Design review of the part built by this model. Coordinates are the model's own, in mm. A direction names the side the tool comes from. Round coordinates to 2 decimals unless told otherwise and drop trailing zeros. Loops run counter-clockwise (first coordinate to the right, second up) from the corner with the lowest first, then second, coordinate; pieces in that order, holes last. Notation, with made-up numbers: (59.25, 39) - (76.25, 39) arc R7 cw to (76.25, 52) - close; hole circle Ø2 at (60, 12). An arc over 180 degrees is marked (long way). One line per question, with ' | ' between items. Start each with the question number.
from build123d import *

# Parameters (mm, degrees)
CROQUIS1_W              = 5.15
CROQUIS1_H              = 40
SALIENTE_EXTRUIR1_DEPTH = 8
CROQUIS2_R              = 1.7
CORTAR_EXTRUIR1_DEPTH   = 11
CROQUIS3_W              = 26
CROQUIS3_H              = 12
CROQUIS3_R              = 4.5
SALIENTE_EXTRUIR2_DEPTH = 5
CROQUIS4_R              = 12
CORTAR_EXTRUIR2_DEPTH   = 1


with BuildPart() as part:
    # Croquis1 → Saliente-Extruir1 (new body)
    with BuildSketch(Plane(origin=(0, 0, 0), x_dir=(1, 0, 0), z_dir=(0, 1, 0))):
        Rectangle(CROQUIS1_W, CROQUIS1_H)
    extrude(amount=-SALIENTE_EXTRUIR1_DEPTH)

    # Croquis2 → Cortar-Extruir1 (cut)
    with BuildSketch(Plane(origin=(2.575, 0, 0), x_dir=(0, 0, -1), z_dir=(1, 0, 0))):
        with Locations((-16, -4)):
            Circle(CROQUIS2_R)
        with Locations((16, -4)):
            Circle(CROQUIS2_R)
    extrude(amount=-CORTAR_EXTRUIR1_DEPTH, mode=Mode.SUBTRACT)

    # Croquis3 → Saliente-Extruir2 (add)
    with BuildSketch(Plane(origin=(0, -8, 0), x_dir=(1, 0, 0), z_dir=(0, 1, 0))):
        with Locations((15.575, 0)):
            Rectangle(CROQUIS3_W, CROQUIS3_H)
        with Locations((15.575, 0)):
            Circle(CROQUIS3_R, mode=Mode.SUBTRACT)
    extrude(amount=SALIENTE_EXTRUIR2_DEPTH)

    # Croquis4 → Cortar-Extruir2 (cut)
    with BuildSketch(Plane(origin=(0, 0, 0), x_dir=(1, 0, 0), z_dir=(0, 1, 0))):
        with Locations((13, 0)):
            Circle(CROQUIS4_R)
    extrude(amount=-CORTAR_EXTRUIR2_DEPTH, mode=Mode.SUBTRACT)


solid = part.part
1. Take a section at B-B, the plane y = -4. Give the boundary of the cut face in (x, z) (3 decimals).
2. Take a section at A-A, the plane z = 16. Give the boundary of the cut face in (x, y) (3 decimals).
3. Machinability: for faces 1 (the face through (15, -6, -6)), 2 (the face through (1, -0.5, -0.1)), 3 (the face through (18, -3, -4)), which of the approach directions +Z, -Z, +X, -X, +Y, -Y give a long, thin tool a straight path to every point of the face, cutting with its end or side? Answer none if there is none.
4. To check wall thickness, follow line 1 along Y through (x, z) = (0, -16); line 2 along X through (y, z) = (-4.3, 0) (3 decimals); line 3 along X through (y, z) = (-1.5, 11) (3 decimals). State the ranges of each line that lie inside material, in increasing order.
5. The part is to be moulded in two halves that separate along Z. For faces 4 (the face through (0, -4, -20)), 5 (the face through (0.04, -4.65, 14.43)), 6 (the face through (28.575, -6, 0)), 7 (the face through (15, -6, 6)), say which applies: pulls with the +Z half, pulls with the -Z half, needs draft (parallel to the pull), parting line crosses it, or undercut.
6. Take a section at C-C, the plane x = 13. Give the boundary of the cut face in (y, z), then the cut area to 3 significant figures.
7. Take a section at D-D, the plane y = -7. Give the boundary of the cut face in (x, z) (3 decimals).
8. Clearance check with flat-ended pins moving along their axes: P1, Ø3, axis at x = 11.5, y = -2.5, coming from the -Z side; P2, Ø4.5, axis at y = -4, z = 16, coming from the +X side (3 decimals); P3, Ø12, axis at x = 20.5, z = 10, coming from the -Y side; P4, Ø3.5, axis at x = 17, z = -2.5, coming from the +Y side. State where each tip first meets the part, or that it passes through.
Answer list:
1) outline: (-2.575, -20) - (2.575, -20) - (2.575, -17.7) - (-2.575, -17.7) - close; (-2.575, -14.3) - (2.575, -14.3) - (2.575, -6) - (28.575, -6) - (28.575, 6) - (2.575, 6) - (2.575, 14.3) - (-2.575, 14.3) - close; (-2.575, 17.7) - (2.575, 17.7) - (2.575, 20) - (-2.575, 20) - close; hole circle Ø9 at (15.575, 0)
2) outline: (-2.575, -8) - (2.575, -8) - (2.575, -5.7) - (-2.575, -5.7) - close; (-2.575, -2.3) - (2.575, -2.3) - (2.575, 0) - (-2.575, 0) - close
3) face 1: -Z, +X, +Y, -Y | face 2: +X, +Y | face 3: +Z, -Z, +X, +Y
4) line 1: y = -8 to -5.7, -2.3 to 0 | line 2: x = -2.575 to 11.075, 20.075 to 28.575 | line 3: x = -2.575 to 2.575
5) face 4: pulls with the -Z half | face 5: undercut | face 6: needs draft | face 7: pulls with the +Z half
6) outline: (-8, -6) - (-3, -6) - (-3, -3.69) - (-8, -3.69) - close; (-8, 3.69) - (-3, 3.69) - (-3, 6) - (-8, 6) - close | area: 23.1 mm²
7) outline: (-2.575, -20) - (2.575, -20) - (2.575, -6) - (28.575, -6) - (28.575, 6) - (2.575, 6) - (2.575, 20) - (-2.575, 20) - close; hole circle Ø9 at (15.575, 0)
8) P1: stops at z = -6 | P2: stops at x = 2.575 | P3: stops at y = -8 | P4: stops at y = -3
